Check sheet for the drawn part. Datum: minimum x, y, z corner. Units: mm. A direction names the side the tool comes from. Give positions to 0.01 mm unless a question says otherwise; leave off trailing zeros. Order: outer loops, then holes, each group sorted by start corner. A loop starts at its lowest first (then second) coordinate and runs counter-clockwise, first axis right, second up. Notation, with made-up numbers: M 82,17.25 L 141,17.25 A16 ccw 141,46.25 Z; hole C 54.5,59.5 d1. An arc over 180 degrees is marked long. Answer in a Markdown table with one row per item. Add a question column.
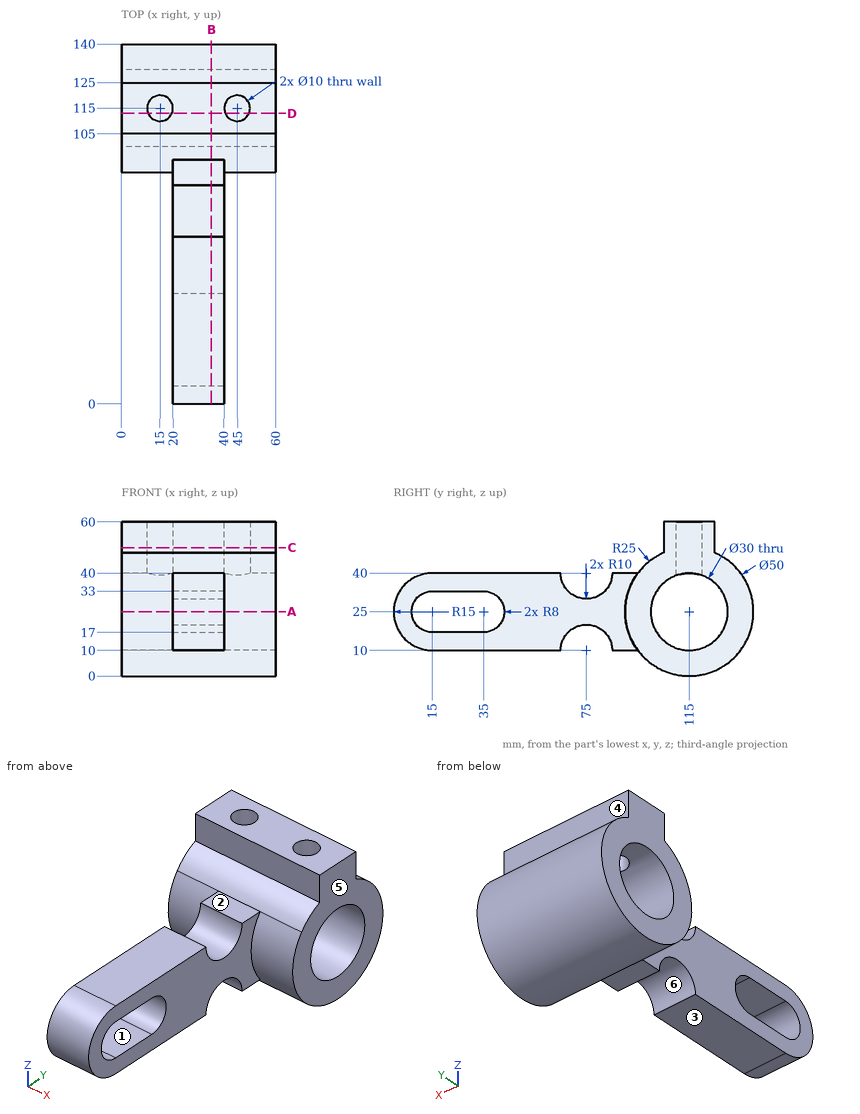
Q1. Tool access check on the marked faces 1, 2 and 3. Record the directions out of +Z, -Z, +X, -X, +Y, -Y that give a thin tool (end or side, any length) a straight path to the whole face; none if there is none.
Q2. Go/stop test with flat-tipped pins: pin 1 (4 mm diameter, centred on x = 27, y = 78.5, fed in from -Z); pin 2 (3 mm diameter, centred on x = 45.5, z = 12.5, fed in from -Y); pin 3 (6 mm diameter, centred on x = 10.5, y = 125, fed in from -Z). Record where each tip stops, or that it passes through.
Q3. Cross-section at D-D (y = 113). Record the boundary of the cut face in (x, z), and give its area (3 significant figures).
Q4. Cross-section at C-C (z = 50). Record the boundary of the cut face in (x, y).
Q5. Draft check along Y on the marked faces 4, 5 and 6. Enter one of: pulls with the +Y half, pulls with the -Y half, needs draft (parallel to the pull), parting line crosses it, or undercut.
Q6. Cross-section at A-A (z = 25). Record the boundary of the cut face in (x, y), and give its area (3 significant figures).
Q7. Thickness scan on probe 1 along Z at (x, y) = (30, 25.5); probe 2 along X at (y, z) = (115, 47.5); probe 3 along Z at (x, y) = (25, 115). Record the ranges inside material, lowest first.
Q8. Cross-section at B-B (x = 35). Record the boundary of the cut face in (y, z).
Values follow:
| question | item | result |
|---|---|---|
| 1 | face 1 | +X, -X |
| 1 | face 2 | +Z, +X, -X, -Y |
| 1 | face 3 | -Z, +X, -X, -Y |
| 2 | pin 1 | z = 18.35 |
| 2 | pin 2 | y = 92.55 |
| 2 | pin 3 | z = 1 |
| 3 | outline | M 0,0.08 L 60,0.08 L 60,10.13 L 0,10.13 Z; M 0,39.87 L 10.42,39.87 L 10.42,60 L 0,60 Z; M 19.58,39.87 L 40.42,39.87 L 40.42,60 L 19.58,60 Z; M 49.58,39.87 L 60,39.87 L 60,60 L 49.58,60 Z |
| 3 | area | 1,440 mm² |
| 4 | outline | M 0,105 L 60,105 L 60,125 L 0,125 Z; hole C 15,115 d10; hole C 45,115 d10 |
| 5 | face 4 | pulls with the +Y half |
| 5 | face 5 | needs draft |
| 5 | face 6 | undercut |
| 6 | outline | M 0,90 L 20,90 L 20,43 L 40,43 L 40,90 L 60,90 L 60,100 L 0,100 Z; M 0,130 L 60,130 L 60,140 L 0,140 Z; M 20,0 L 40,0 L 40,7 L 20,7 Z |
| 6 | area | 2,280 mm² |
| 7 | probe 1 | 10 to 17, 33 to 40 |
| 7 | probe 2 | 0 to 10, 20 to 40, 50 to 60 |
| 7 | probe 3 | 0 to 10, 40 to 60 |
| 8 | outline | M 15,10 L 65,10 A10 cw 85,10 L 95,10 A25 ccw long 125,47.91 L 125,60 L 105,60 L 105,47.91 A25 ccw 95,40 L 85,40 A10 cw 65,40 L 15,40 A15 ccw Z; hole M 15,17 L 35,17 A8 ccw 35,33 L 15,33 A8 ccw Z; hole C 115,25 d30 |
